For this review, take the finished solid that the model builds, in its own axes (mm). Face numbers are marked on the shaded views. A direction names the side the tool comes from. Give positions to 0.01 mm unless a question says otherwise; leave off trailing zeros. Loops run counter-clockwise (first coordinate to the right, second up) from the corner with the lowest first, then second, coordinate; pieces in that order, holes last. Notation, with made-up numbers: (72, 38) - (98, 38) arc R21 cw to (98, 48) - close; hole circle Ø3 at (-12, 50). An arc over 180 degrees is marked (long way). Answer in a Markdown table with one row per item.
```python
from build123d import *

# Parameters (mm, degrees)
SKETCH004_R           = 32
SKETCH004_R_2         = 30
PAD002_DEPTH          = 40
SKETCH005_R           = 30
SKETCH005_R_2         = 28
PAD003_DEPTH          = 30
CHAMFER_SIZE          = 1.9
CHAMFER001_SIZE       = 1.9
REVOLUTION_ANGLE      = 10
POLARPATTERN_COUNT    = 8
SKETCH007_W           = 15
SKETCH007_H           = 5
SKETCH007_W_2         = 13
REVOLUTION001_ANGLE   = 10
POLARPATTERN001_COUNT = 6
SKETCH009_R           = 45
SKETCH009_R_2         = 43
PAD004_DEPTH          = 30
SKETCH010_W           = 80
SKETCH010_H           = 80
SKETCH010_R           = 32
PAD005_DEPTH          = 3
SKETCH011_R           = 3
POCKET002_DEPTH       = 3
FILLET001_R           = 6
SKETCH021_R           = 30.5
POCKET004_DEPTH       = 27


with BuildPart() as part:
    # Sketch004 → Pad002 (new body)
    with BuildSketch(Plane.XY):
        Circle(SKETCH004_R)
        Circle(SKETCH004_R_2, mode=Mode.SUBTRACT)
    extrude(amount=PAD002_DEPTH)

    # Sketch005 (on Face4 of Pad002) → Pad003 (join)
    with BuildSketch(Plane.XY.offset(27)):
        Circle(SKETCH005_R)
        Circle(SKETCH005_R_2, mode=Mode.SUBTRACT)
    extrude(amount=PAD003_DEPTH)

    # Chamfer
    chamfer_edges = [part.edges().sort_by_distance(p)[0] for p in [
        (-32, 0, 40),
    ]]
    chamfer(chamfer_edges, length=CHAMFER_SIZE)

    # Chamfer001
    chamfer001_edges = [part.edges().sort_by_distance(p)[0] for p in [
        (-28, 0, 27),
    ]]
    chamfer(chamfer001_edges, length=CHAMFER001_SIZE)

    # Sketch006 → Revolution (revolve)
    with BuildSketch(Plane.YZ):
        Polygon((-28, 40), (-28, 48.660254), (-23, 48.660254), align=None)
    revolution = revolve(axis=Axis((0, 0, 0), (0, 0, 1)), revolution_arc=REVOLUTION_ANGLE)

    # PolarPattern: Revolution ×8 about axis
    polarpattern_axis = Axis((0, 0, 0), (0, 0, 1))
    for i in range(1, POLARPATTERN_COUNT):
        add(revolution.rotate(polarpattern_axis, i * 360 / POLARPATTERN_COUNT))

    # Sketch007 → Revolution001 (revolve)
    with BuildSketch(Plane.YZ):
        with Locations((-37.5, 54.5)):
            Rectangle(SKETCH007_W, SKETCH007_H)
        with Locations((-38.5, 29.5)):
            Rectangle(SKETCH007_W_2, SKETCH007_H)
    revolution001 = revolve(axis=Axis((0, 0, 0), (0, 0, 1)), revolution_arc=REVOLUTION001_ANGLE)

    # PolarPattern001: Revolution001 ×6 about axis
    polarpattern001_axis = Axis((0, 0, 0), (0, 0, 1))
    for i in range(1, POLARPATTERN001_COUNT):
        add(revolution001.rotate(polarpattern001_axis, i * 360 / POLARPATTERN001_COUNT))

    # Sketch008 → Revolution002 (revolve)
    with BuildSketch(Plane.YZ):
        Polygon((-45, 57), (0, 94.759483), (0, 93.081284), (-43, 57), align=None)
    revolve(axis=Axis((0, 0, 0), (0, 0, 1)))

    # Sketch009 (on Face100 of Revolution002) → Pad004 (join)
    with BuildSketch(Plane(origin=(0, 0, 57), x_dir=(1, 0, 0), z_dir=(0, 0, -1))):
        Circle(SKETCH009_R)
        Circle(SKETCH009_R_2, mode=Mode.SUBTRACT)
    extrude(amount=PAD004_DEPTH)

    # Sketch010 (on Face5 of Pad004) → Pad005 (join)
    with BuildSketch(Plane(origin=(0, 0, 0), x_dir=(1, 0, 0), z_dir=(0, 0, -1))):
        Rectangle(SKETCH010_W, SKETCH010_H)
        Circle(SKETCH010_R, mode=Mode.SUBTRACT)
    extrude(amount=-PAD005_DEPTH)

    # Sketch011 (on Face39 of Pad005) → Pocket002 (cut)
    with BuildSketch(Plane(origin=(0, 0, 0), x_dir=(1, 0, 0), z_dir=(0, 0, -1))):
        with Locations((-30, 30)):
            Circle(SKETCH011_R)
        with Locations((30, 30)):
            Circle(SKETCH011_R)
        with Locations((-30, -30)):
            Circle(SKETCH011_R)
        with Locations((30, -30)):
            Circle(SKETCH011_R)
    extrude(amount=-POCKET002_DEPTH, mode=Mode.SUBTRACT)

    # Fillet001
    fillet001_edges = [part.edges().sort_by_distance(p)[0] for p in [
        (40, 40, 1.5),
        (-40, 40, 1.5),
        (-40, -40, 1.5),
        (40, -40, 1.5),
    ]]
    fillet(fillet001_edges, radius=FILLET001_R)

    # Sketch021 (on Face1 of Fillet001) → Pocket004 (cut)
    with BuildSketch(Plane(origin=(0, 0, 0), x_dir=(1, 0, 0), z_dir=(0, 0, -1))):
        Circle(SKETCH021_R)
    extrude(amount=-POCKET004_DEPTH, mode=Mode.SUBTRACT)


with BuildPart() as part_1:
    # Body001 placement: moved
    add(part.part.moved(Location((0, 0, 3))))


solid = part_1.part
```
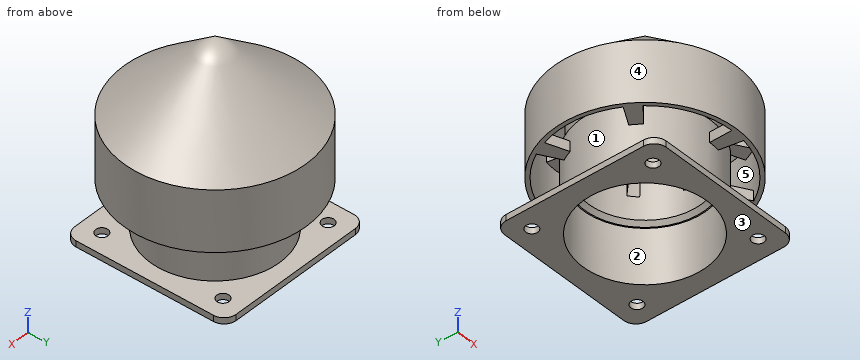
1. Clearance check with flat-ended pins moving along their axes: pin 1 (6 mm diameter, centred on y = 21.5, z = 63, fed in from +X); pin 2 (5.5 mm diameter, centred on y = -38, z = 57, fed in from -X); pin 3 (6 mm diameter, centred on x = 3.5, y = -36, fed in from +Z). State where each tip first meets the part, or that it passes through.
Values:
| item | result |
|---|---|
| pin 1 | stops at x = 39.83 |
| pin 2 | stops at x = -27.97 |
| pin 3 | stops at z = 69.93 |
2. For the marked faces 4 and 5, list the 3-axis set-ups (+Z, -Z, +X, -X, +Y, -Y) from which the entire face can be reached by the end or side of a thin tool; tool diameter is ignored.
Values:
| item | result |
|---|---|
| face 4 | +Z |
| face 5 | none |
3. Mouldability with a two-part tool opening along Z and no side actions: class the marked faces 1, 2 and 3 as released by +Z, released by -Z, zero draft, split by the parting line, or undercut.
Values:
| item | result |
|---|---|
| face 1 | undercut |
| face 2 | zero draft |
| face 3 | released by -Z |
4. We need section A-A, the plane y = -25. Count the separate pieces of the cut face and the enclosed holes in it, and give its area (3 significant figures).
Values:
| item | result |
|---|---|
| separate pieces | 4 |
| enclosed holes | 0 |
| area | 904 mm^2 |
5. Wall thickness on line 1 (Y direction, x = -19, z = 44); line 2 (Y direction, x = 5.5, z = 30.5); line 3 (X direction, y = 0, z = 12): over which ranges is each line inside the solid? List them lowest first. Write a range as [from, to].
Values:
| item | result |
|---|---|
| line 1 | y = [-40.79, -38.57], [-23.22, -19.77], [20.57, 23.22], [38.57, 40.79] |
| line 2 | y = [-44.66, -28.88], [28.88, 31.52], [42.65, 44.66] |
| line 3 | x = [-32, -30.5], [30.5, 32] |
6. We need section B-B, the plane z = 86.5. Give the boundary of the cut face in (x, y), and give its area (3 significant figures).
Values:
| item | result |
|---|---|
| outline | circle Ø26.84 at (0, 0); hole circle Ø22.84 at (0, 0) |
| area | 156 mm^2 |
